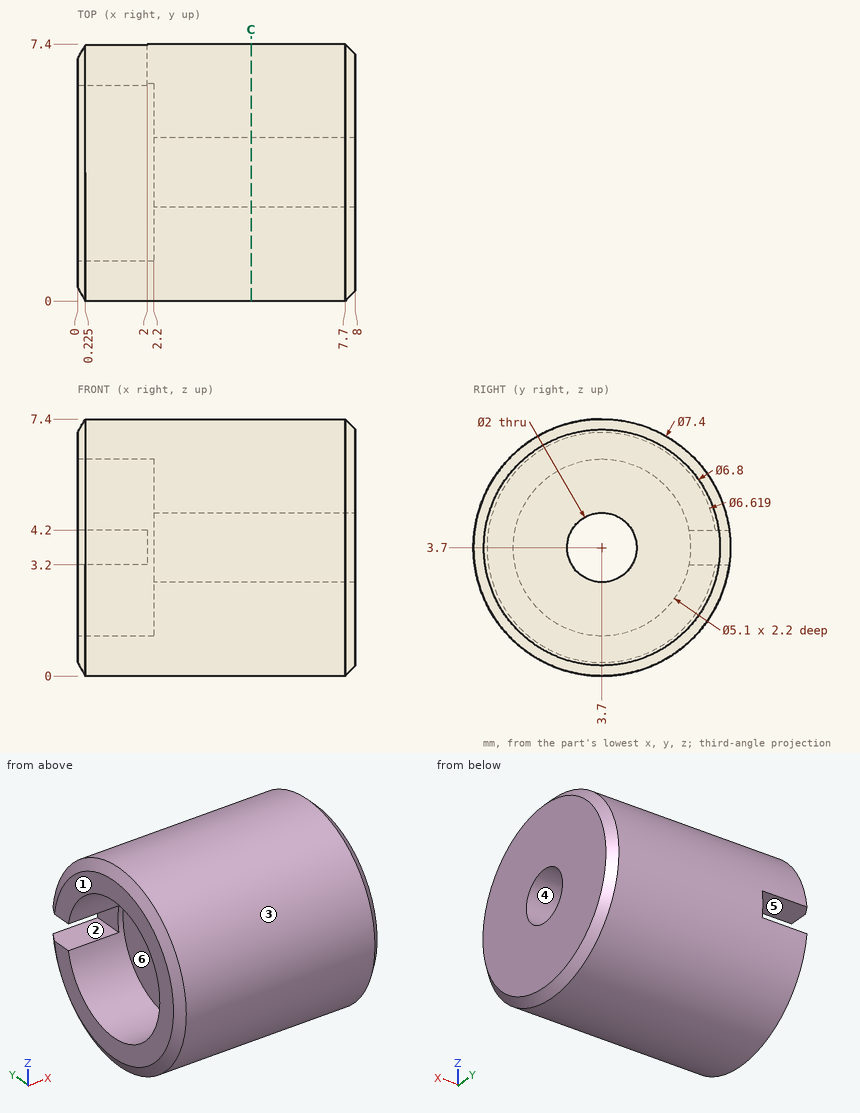
Can you work these out from the drawing? Everything is in mm from the part's minimum corner. A direction names the side the tool comes from. Give positions to 0.01 mm unless a question says otherwise; leave off trailing zeros. Order: outer loops, then holes, each group sorted by start corner. A loop starts at its lowest first (then second) coordinate and runs counter-clockwise, first axis right, second up. Notation, with made-up numbers: M 65,2 L 102,2 A16 cw 102,32 Z; hole C -21,57.25 d6. An arc over 180 degrees is marked long. Use a Markdown table: item, result. Add a question column.
Item 1: For the marked faces 4, 5 and 6, which set-ups out of +Z, -Z, +X, -X, +Y, -Y let a thin tool reach every point of the face, with its end or its side?
Item 2: We'd pull the mould along Z, two halves only. Please class the marked faces 1, 2 and 3: +Z half, -Z half, draft (parallel to the pull), parting line (faces both ways), or undercut.
Item 3: If I drill on L1, parallel to Y at x = 3.4, z = 3.7; L2, parallel to Z at x = 1.3, y = 3.7; L3, parallel to X at y = 5, z = 4.25, over which ranges is the centre line in solid material (lowest first)? Write a range as [from, to].
Item 4: Will these pins go through, and if not, where does the flat tip stop? pin 1 (1 mm diameter, centred on x = 3.5, z = 1, fed in from +Y) (1 decimal); pin 2 (4 mm diameter, centred on x = 1.5, z = 6, fed in from -Y); pin 3 (2 mm diameter, centred on x = 2, z = 5, fed in from +Y).
Item 5: Suppose I cut it at C-C (x = 5). List the corners of the cut face in (y, z) for me.
Answer sheet:
| question | item | result |
|---|---|---|
| 1 | face 4 | +X, -X |
| 1 | face 5 | -X, +Y |
| 1 | face 6 | -X |
| 2 | face 1 | draft |
| 2 | face 2 | undercut |
| 2 | face 3 | parting line |
| 3 | L1 | y = [0, 2.7], [4.7, 7.4] |
| 3 | L2 | z = [0, 1.15], [6.25, 7.4] |
| 3 | L3 | x = [2.2, 8] |
| 4 | pin 1 | stops at y = 6.7 |
| 4 | pin 2 | stops at y = 0.01 |
| 4 | pin 3 | stops at y = 7.39 |
| 5 | outline | C 3.7,3.7 d7.4; hole C 3.7,3.7 d2 |
